The figure shows three views and two pictorial views of one solid part (mm, origin at its lowest corner). Answer the questions. A direction names the side the tool comes from. Round coordinates to 2 decimals unless told otherwise and drop trailing zeros. Order: outer loops, then holes, each group sorted by start corner. A loop starts at its lowest first (then second) coordinate and runs counter-clockwise, first axis right, second up.
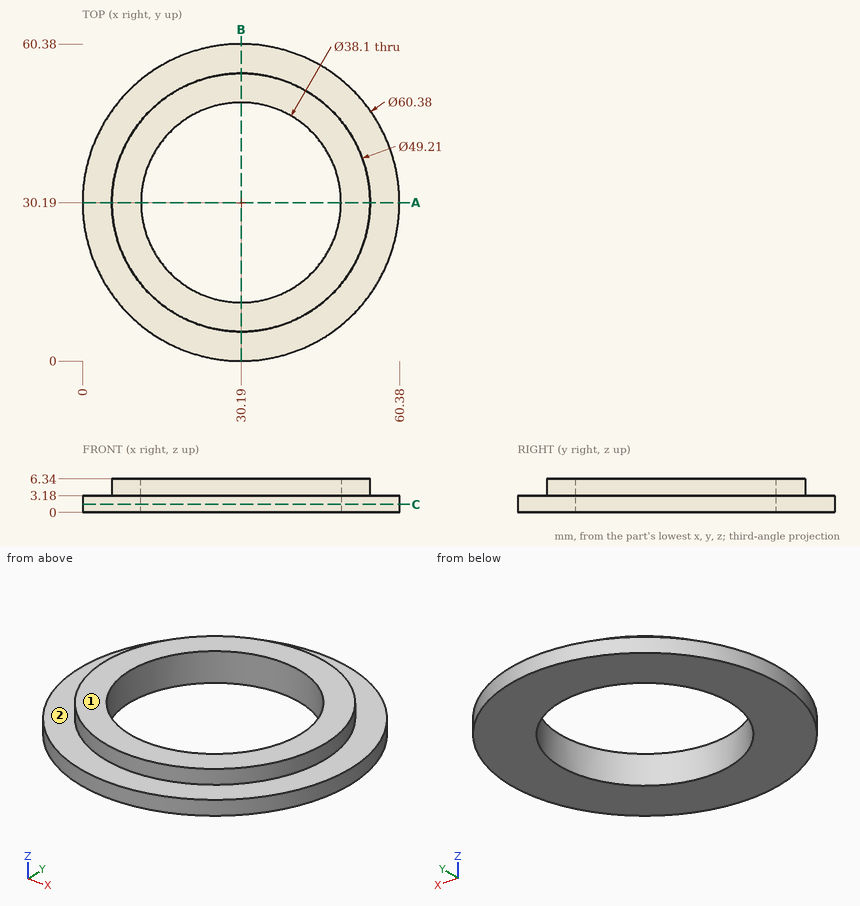
Item 1: A tool of negligible diameter and unlimited length cuts with its end or side. For the marked faces 1 and 2, from which of +Z, -Z, +X, -X, +Y, -Y can it reach the whole face along a straight path? Write none if from no direction.
Item 2: Find section C-C (z = 1.5). Write down the section's boundary in (x, y).
Item 3: Find the intervals of material crossed by line 1 along Y through (x, z) = (30.19, 2); line 2 along Y through (x, z) = (30.19, 4.5) (3 decimals); line 3 along X through (y, z) = (12.5, 5), in increasing order.
Item 4: Find section A-A (y = 30.19). Write down the section's boundary in (x, z) (3 decimals).
Item 5: Given pin 1 (1 mm diameter, centred on x = 31, z = 0.5, fed in from -Y), flat-ended and moving along its own axis, determine where the tip first touches the part or whether it passes through.
Model answer:
1. face 1: +Z, +X, -X, +Y, -Y
1. face 2: +Z
2. outline: circle Ø60.38 at (30.19, 30.19); hole circle Ø38.1 at (30.19, 30.19)
3. line 1: y = 0 to 11.14, 49.24 to 60.38
3. line 2: y = 5.585 to 11.14, 49.24 to 54.795
3. line 3: x = 13.09 to 23.12, 37.26 to 47.29
4. outline: (0, 0) - (11.14, 0) - (11.14, 6.34) - (5.585, 6.34) - (5.585, 3.18) - (0, 3.18) - close; (49.24, 0) - (60.38, 0) - (60.38, 3.18) - (54.795, 3.18) - (54.795, 6.34) - (49.24, 6.34) - close
5. pin 1: stops at y = 0
